Source: CAD feature listing. Evaluate the final solid. Frame: model axes, mm. A direction names the side the tool comes from. Coordinates: 2 decimals unless noted, no trailing zeros. Write each loop counter-clockwise with the first axis right and the second up, starting at its lowest first coordinate (ties: lowest second). Pieces come first, ordered by that corner, then holes. Notation, with made-up numbers: M -36,-15.75 L -30,-15.75 A17 cw -30,-8.75 Z; hole C 82,72 d1. An arc over 180 degrees is marked long. Answer as CSV lines item,"result". Start each with the question number.
1. Section A-A on y = 69.5. Return the cut outline in (x, z), plus the area to 3 significant figures.
2. Mould query, pull axis X, two halves, no side actions, for faces 1 (the face through (0, 9, 8.5)), 2 (the face through (0, 7.751, 12)), 3 (the face through (0, 7, 15)), 4 (the face through (9.216, 12.882, -0.056)). Classes: pulls with the +X half, pulls with the -X half, needs draft (parallel to the pull), parting line crosses it, or undercut.
3. Section B-B on z = 0. Return the cut outline in (x, y), plus the area to 3 significant figures.
4. Line query: probe 1 along X at (y, z) = (9.5, 11); probe 2 along Y at (x, z) = (0, 11); probe 3 along Z at (x, y) = (8, 13). Output: solid intervals per line, ascending. Write a range as [from, to].
5. Reachability of faces 5 (the face through (0, 90, 0)), 6 (the face through (8, 5, 4)), 7 (the face through (3.417, 53.682, 0.759)) from +Z, -Z, +X, -X, +Y, -Y: full face, straight path, thin tool, end or side. Return the list, or none.
6. Contact query for flat-ended pins moving along their axis: pin 1 Ø1.7 at (x, y) = (-0.5, 9.5) entering from +Z; pin 2 Ø10 at (x, z) = (-1.5, 8.5) entering from +Y; pin 3 Ø3 at (x, z) = (0, 12.5) entering from +Y. Output: stop coordinate, or through.
```python
from build123d import *

# Parameters (mm, degrees)
SKETCH1_R           = 3.5
BOSS_EXTRUDE1_DEPTH = 90
SKETCH4_R           = 10
BOSS_EXTRUDE2_DEPTH = 4
BOSS_EXTRUDE3_START = -4
SKETCH4_7_R         = 10
BOSS_EXTRUDE3_DEPTH = 4
CUT_EXTRUDE3_DEPTH  = 6.5


with BuildPart() as part:
    # Sketch1 → Boss-Extrude1 (new body)
    with BuildSketch(Plane(origin=(0, 0, 0), x_dir=(1, 0, 0), z_dir=(0, 1, 0))):
        with Locations(Location((0, 0, 0), (0, 0, 90))):
            Circle(SKETCH1_R)
    extrude(amount=BOSS_EXTRUDE1_DEPTH)

    # Sketch4 → Boss-Extrude2 (add)
    with BuildSketch(Plane.XY):
        with Locations(Location((0, 9, 0), (0, 0, 110.487315115))):
            Circle(SKETCH4_R)
    extrude(amount=BOSS_EXTRUDE2_DEPTH)

    # Sketch4<7> → Boss-Extrude3 (add)
    with BuildSketch(Plane.XY.offset(BOSS_EXTRUDE3_START)):
        with Locations((0, 9)):
            Circle(SKETCH4_7_R)
    extrude(amount=BOSS_EXTRUDE3_DEPTH)

    # Loft2: read off the stored shape, not the designer's step
    # Loft2: loft between two sections, ruled curve by curve
    loft2_from = [
        Edge.make_bspline([(-9.973450677, 9.728204366, 0), (-11.429859409, -10.218696987, 0), (8.517041945, -11.67510572, 0), (9.973450677, 8.271795634, 0), (11.429859409, 28.218696987, 0), (-8.517041945, 29.67510572, 0), (-9.973450677, 9.728204366, 0)], [0, 0, 0, 0, 0.5, 0.5, 0.5, 1, 1, 1, 1], 3, [1, 0.333333333, 0.333333333, 1, 0.333333333, 0.333333333, 1]),
    ]
    loft2_to = [
        Edge.make_bspline([(-3.898107491, 8.102916956, 15), (-2.103941404, 0.306701974, 15), (5.692273579, 2.100868062, 15), (3.898107491, 9.897083044, 15), (2.103941404, 17.693298026, 15), (-5.692273579, 15.899131938, 15), (-3.898107491, 8.102916956, 15)], [0, 0, 0, 0, 0.5, 0.5, 0.5, 1, 1, 1, 1], 3, [1, 0.333333333, 0.333333333, 1, 0.333333333, 0.333333333, 1]),
    ]
    loft2 = Solid(Shell([*[Face.make_surface_from_curves(loft2_from[k], loft2_to[k]) for k in range(1)], Face(Wire(loft2_from)), Face(Wire(loft2_to))]))
    add(loft2)

    # Sketch5 → Cut-Extrude3 (cut)
    with BuildSketch(Plane.XY.offset(15)):
        with BuildLine():
            Line((1.99219482, 7.750633525), (-1.99219482, 7.750633525))
            ThreePointArc((-1.99219482, 7.750633525), (0, 11.200050682), (1.99219482, 7.750633525))
        make_face()
    extrude(amount=-CUT_EXTRUDE3_DEPTH, mode=Mode.SUBTRACT)


solid = part.part
```
Values:
1,outline,"C 0,0 d7"
1,area,"38.5 mm²"
2,face 1,"undercut"
2,face 2,"undercut"
2,face 3,"needs draft"
2,face 4,"parting line crosses it"
3,outline,"M -3.5,18.37 A10 ccw long 3.5,18.37 L 3.5,90 L -3.5,90 Z"
3,area,"813 mm²"
4,probe 1,"[-5.52, -2.22], [2.22, 5.52]"
4,probe 2,"[3.46, 7.75], [11.2, 14.54]"
4,probe 3,"[-4, 4]"
5,face 5,"+Z, -Z, +X, -X, +Y"
5,face 6,"+Z"
5,face 7,"+Y"
6,pin 1,"z = 8.5"
6,pin 2,"y = 19"
6,pin 3,"y = 14.54"
